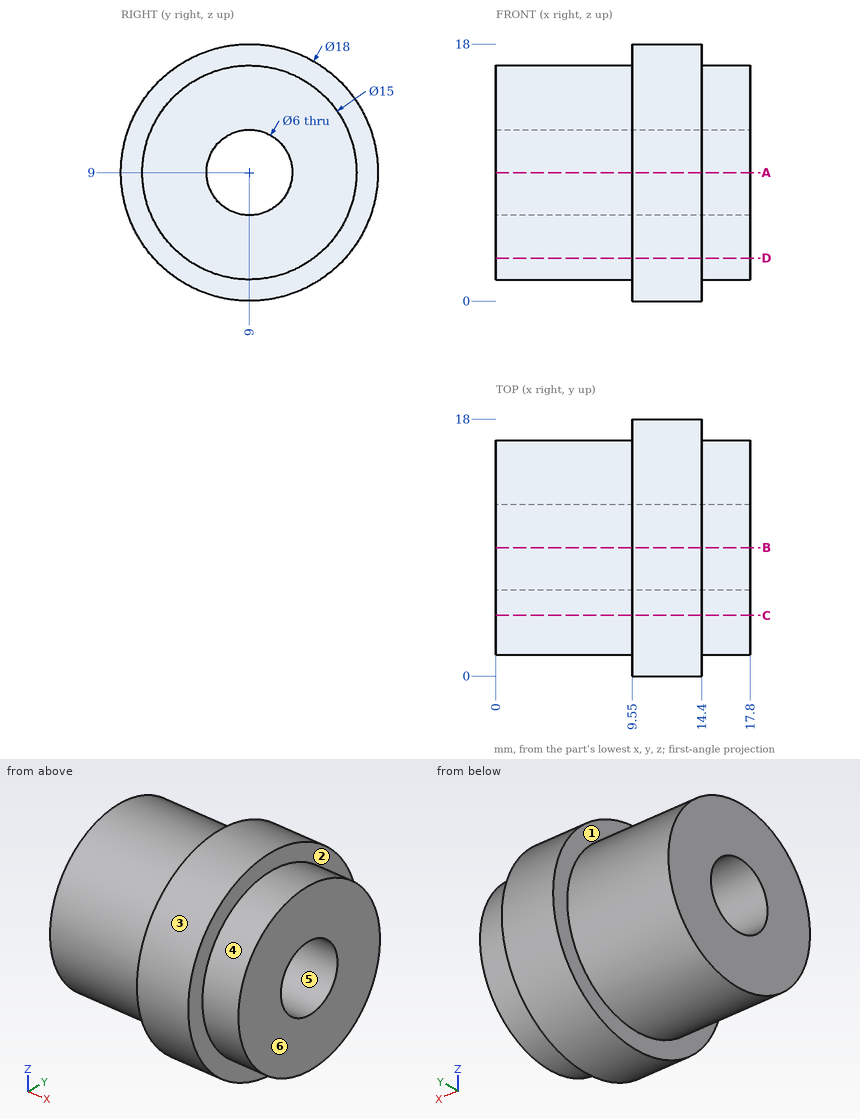
Design review of the part shown in the three views and the two pictorial views. Dimensions are in mm from the part's minimum x, y and z. A direction names the side the tool comes from. Round coordinates to 2 decimals unless told otherwise and drop trailing zeros. Loops run counter-clockwise (first coordinate to the right, second up) from the corner with the lowest first, then second, coordinate; pieces in that order, holes last. Notation, with made-up numbers: (24, 42) -> (32, 42) arc R21 cw to (32, 71) -> close; hole circle Ø2 at (-31, 27). An arc over 180 degrees is marked (long way). Use one line per item in the form item = value. Start each with the question number.
Q1. We need section A-A on z = 9. Give the boundary of the cut face in (x, y).
Q2. We need section C-C on y = 4.25. Give the boundary of the cut face in (x, z).
Q3. Machinability: for the marked faces 1, 2 and 3, which of the approach directions +Z, -Z, +X, -X, +Y, -Y give a long, thin tool a straight path to every point of the face, cutting with its end or side? Answer none if there is none.
Q4. For pin 1 Ø2 at (x, y) = (13, 8) entering from -Z; pin 2 Ø2 at (x, y) = (5.5, 13) entering from +Z; pin 3 Ø4 at (x, y) = (3, 6) entering from -Z; pin 4 Ø3 at (x, y) = (11, 4) entering from -Z, all flat-tipped, find the tip position at first contact; note any pin that passes through.
Q5. Wall thickness on line 1 along Y through (x, z) = (12, 9); line 2 along Y through (x, z) = (9, 9); line 3 along X through (y, z) = (1, 13): over which ranges is each line inside the solid? List them lowest first. Write a range as [from, to].
Q6. We need section D-D on z = 3. Give the boundary of the cut face in (x, y).
Q7. Draft analysis for pull direction Y (two halves, no side actions). For the marked faces 4, 5 and 6, state which applies: +Y half, -Y half, draft (parallel to the pull), parting line (faces both ways), or undercut.
Calculated:
q1.outline = (0, 1.5) -> (9.55, 1.5) -> (9.55, 0) -> (14.4, 0) -> (14.4, 1.5) -> (17.8, 1.5) -> (17.8, 6) -> (0, 6) -> close; (0, 12) -> (17.8, 12) -> (17.8, 16.5) -> (14.4, 16.5) -> (14.4, 18) -> (9.55, 18) -> (9.55, 16.5) -> (0, 16.5) -> close
q2.outline = (0, 3.2) -> (9.55, 3.2) -> (9.55, 1.36) -> (14.4, 1.36) -> (14.4, 3.2) -> (17.8, 3.2) -> (17.8, 14.8) -> (14.4, 14.8) -> (14.4, 16.64) -> (9.55, 16.64) -> (9.55, 14.8) -> (0, 14.8) -> close
q3.face_1 = -X
q3.face_2 = +X
q3.face_3 = +X, -X
q4.pin_1 = 0
q4.pin_2 = 15.87
q4.pin_3 = 1.57
q4.pin_4 = 0.71
q5.line_1 = [0, 6], [12, 18]
q5.line_2 = [1.5, 6], [12, 16.5]
q5.line_3 = [9.55, 14.4]
q6.outline = (0, 4.5) -> (9.55, 4.5) -> (9.55, 2.29) -> (14.4, 2.29) -> (14.4, 4.5) -> (17.8, 4.5) -> (17.8, 13.5) -> (14.4, 13.5) -> (14.4, 15.71) -> (9.55, 15.71) -> (9.55, 13.5) -> (0, 13.5) -> close
q7.face_4 = parting line
q7.face_5 = undercut
q7.face_6 = draft
